```python
from build123d import *

# Parameters (mm, degrees)
SALIENTE_EXTRUIR1_DEPTH = 10
CROQUIS2_R              = 4.25
CORTAR_EXTRUIR1_DEPTH   = 11
CROQUIS3_R              = 4.25
CORTAR_EXTRUIR2_DEPTH   = 11


with BuildPart() as part:
    # Croquis1 → Saliente-Extruir1 (new body)
    with BuildSketch(Plane.XY):
        Polygon((-300, 0), (-250, 0), (-250, 50), (-50, 50), (-50, 0), (0, 0), (0, 300), (-300, 300), align=None)
    extrude(amount=SALIENTE_EXTRUIR1_DEPTH)

    # Croquis2 → Cortar-Extruir1 (cut, through all)
    with BuildSketch(Plane.XY.offset(10)):
        with Locations((-280, 25)):
            Circle(CROQUIS2_R)
        with Locations((-280, 277)):
            Circle(CROQUIS2_R)
        with Locations((-80, 277)):
            Circle(CROQUIS2_R)
        with Locations((-220, 277)):
            Circle(CROQUIS2_R)
        with Locations((-20, 277)):
            Circle(CROQUIS2_R)
        with Locations((-20, 25)):
            Circle(CROQUIS2_R)
        with Locations((120, 277)):
            Circle(CROQUIS2_R)
        with Locations((-420, 277)):
            Circle(CROQUIS2_R)
    extrude(amount=-CORTAR_EXTRUIR1_DEPTH, mode=Mode.SUBTRACT)

    # Croquis3 → Cortar-Extruir2 (cut, through all)
    with BuildSketch(Plane.XY.offset(10)):
        with Locations((-100, 85)):
            Circle(CROQUIS3_R)
        with Locations((-350, 85)):
            Circle(CROQUIS3_R)
        with Locations((-475, 85)):
            Circle(CROQUIS3_R)
        with Locations((50, 85)):
            Circle(CROQUIS3_R)
        with Locations((-200, 85)):
            Circle(CROQUIS3_R)
    extrude(amount=-CORTAR_EXTRUIR2_DEPTH, mode=Mode.SUBTRACT)


solid = part.part
```
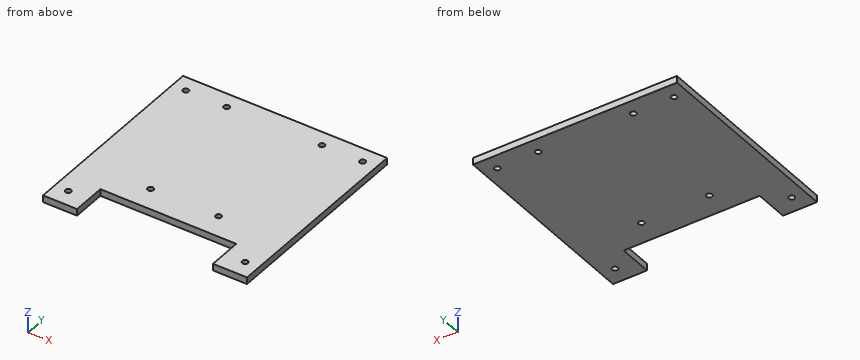
Can you work these out from the model? Positions are in its coordinate system, mm. Round coordinates to 2 decimals unless told otherwise and drop trailing zeros. Loops run counter-clockwise (first coordinate to the right, second up) from the corner with the lowest first, then second, coordinate; pieces in that order, holes last. Notation, with made-up numbers: M 9,39 L 53,39 A17 ccw 53,51 Z; hole C 57,60.5 d8. An arc over 180 degrees is marked long. Answer in a Markdown table with one row per item.
1. Please list where these lines run through material, in increasing order: line 1 (X direction, y = 46, z = 3); line 2 (Y direction, x = -220, z = 7); line 3 (Y direction, x = -120, z = 7). Write a range as from..to.
Established:
| item | result |
|---|---|
| line 1 | -300..-250, -50..0 |
| line 2 | 50..272.75, 281.25..300 |
| line 3 | 50..300 |
2. If we section it at C-C, the plane x = -100: Please give me the cut outline in (y, z), plus the area to 4 significant figures.
Established:
| item | result |
|---|---|
| outline | M 50,0 L 80.75,0 L 80.75,10 L 50,10 Z; M 89.25,0 L 300,0 L 300,10 L 89.25,10 Z |
| area | 2,415 mm² |
3. I'm going to push a flat-ended pin straight in: pin 1 Ø1 at (x, z) = (-176.5, 8.5) entering from -Y. Where does the tip first touch, or does it pass through?
Established:
| item | result |
|---|---|
| pin 1 | y = 50 |
4. If we section it at B-B, the plane x = -280: Please give me the cut outline in (y, z), plus the area to 3 significant figures.
Established:
| item | result |
|---|---|
| outline | M 0,0 L 20.75,0 L 20.75,10 L 0,10 Z; M 29.25,0 L 272.75,0 L 272.75,10 L 29.25,10 Z; M 281.25,0 L 300,0 L 300,10 L 281.25,10 Z |
| area | 2,830 mm² |
5. If we section it at D-D, the plane z = 1.75: Give the number of separate pieces and of enclosed holes in the cut face, plus the area to 3 significant figures.
Established:
| item | result |
|---|---|
| separate pieces | 1 |
| enclosed holes | 8 |
| area | 79,500 mm² |
6. If we section it at A-A, the plane y = 85: Please give me the cut outline in (x, z), plus the area to 3 significant figures.
Established:
| item | result |
|---|---|
| outline | M -300,0 L -204.25,0 L -204.25,10 L -300,10 Z; M -195.75,0 L -104.25,0 L -104.25,10 L -195.75,10 Z; M -95.75,0 L 0,0 L 0,10 L -95.75,10 Z |
| area | 2,830 mm² |
